```python
from build123d import *

# Parameters (mm, degrees)
CELL_BLOCK_SKETCH_W = 162.5
CELL_BLOCK_SKETCH_H = 305.12867922
BOSS_EXTRUDE1_DEPTH = 5
SKETCH3_W           = 7.5
SKETCH3_H           = 305.12867922
BOSS_EXTRUDE2_DEPTH = 5
HOLE_PATTERN_R      = 10.875
CUT_EXTRUDE1_DEPTH  = 5
SKETCH4_R           = 3.3
CUT_EXTRUDE2_DEPTH  = 5
SKETCH5_W           = 152.5
SKETCH5_H           = 25
BOSS_EXTRUDE3_DEPTH = 5
FILLET1_R           = 20


with BuildPart() as part:
    # Cell Block Sketch → Boss-Extrude1 (new body)
    with BuildSketch(Plane(origin=(0, 0, 0), x_dir=(1, 0, 0), z_dir=(0, 1, 0))):
        Rectangle(CELL_BLOCK_SKETCH_W, CELL_BLOCK_SKETCH_H)
    extrude(amount=BOSS_EXTRUDE1_DEPTH)

    # Sketch3 → Boss-Extrude2 (add)
    with BuildSketch(Plane(origin=(0, 0, 0), x_dir=(1, 0, 0), z_dir=(0, 1, 0))):
        with Locations((-85, 0)):
            Rectangle(SKETCH3_W, SKETCH3_H)
    boss_extrude2 = extrude(amount=BOSS_EXTRUDE2_DEPTH)

    # Mirror1: Boss-Extrude2 across plane
    add(boss_extrude2.mirror(Plane(origin=(0, 0, 0), x_dir=(0, 0, 1), z_dir=(1, 0, 0))))

    # Hole Pattern → Cut-Extrude1 (cut)
    with BuildSketch(Plane(origin=(0, 5, 0), x_dir=(1, 0, 0), z_dir=(0, 1, 0))):
        with Locations(Location((-70.375, -111.814056593, 0), (0, 0, 270))):
            Circle(HOLE_PATTERN_R)
        with Locations(Location((-58.9, -131.68933961, 0), (0, 0, 270))):
            Circle(HOLE_PATTERN_R)
        with Locations(Location((-70.375, -72.063490559, 0), (0, 0, 270))):
            Circle(HOLE_PATTERN_R)
        with Locations(Location((-58.9, -91.938773576, 0), (0, 0, 270))):
            Circle(HOLE_PATTERN_R)
        with Locations(Location((-70.375, -32.312924525, 0), (0, 0, 270))):
            Circle(HOLE_PATTERN_R)
        with Locations(Location((-58.9, -52.188207542, 0), (0, 0, 270))):
            Circle(HOLE_PATTERN_R)
        with Locations(Location((-70.375, 7.437641508, 0), (0, 0, 270))):
            Circle(HOLE_PATTERN_R)
        with Locations(Location((-58.9, -12.437641508, 0), (0, 0, 270))):
            Circle(HOLE_PATTERN_R)
        with Locations(Location((-70.375, 47.188207542, 0), (0, 0, 270))):
            Circle(HOLE_PATTERN_R)
        with Locations(Location((-58.9, 27.312924525, 0), (0, 0, 270))):
            Circle(HOLE_PATTERN_R)
        with Locations(Location((-70.375, 86.938773576, 0), (0, 0, 270))):
            Circle(HOLE_PATTERN_R)
        with Locations(Location((-58.9, 67.063490559, 0), (0, 0, 270))):
            Circle(HOLE_PATTERN_R)
        with Locations(Location((-70.375, 126.68933961, 0), (0, 0, 270))):
            Circle(HOLE_PATTERN_R)
        with Locations(Location((-58.9, 106.814056593, 0), (0, 0, 270))):
            Circle(HOLE_PATTERN_R)
        with Locations(Location((-47.425, -72.063490559, 0), (0, 0, 270))):
            Circle(HOLE_PATTERN_R)
        with Locations(Location((-35.95, -91.938773576, 0), (0, 0, 270))):
            Circle(HOLE_PATTERN_R)
        with Locations(Location((-47.425, -32.312924525, 0), (0, 0, 270))):
            Circle(HOLE_PATTERN_R)
        with Locations(Location((-35.95, -52.188207542, 0), (0, 0, 270))):
            Circle(HOLE_PATTERN_R)
        with Locations(Location((-47.425, 7.437641508, 0), (0, 0, 270))):
            Circle(HOLE_PATTERN_R)
        with Locations(Location((-35.95, -12.437641508, 0), (0, 0, 270))):
            Circle(HOLE_PATTERN_R)
        with Locations(Location((-47.425, 47.188207542, 0), (0, 0, 270))):
            Circle(HOLE_PATTERN_R)
        with Locations(Location((-35.95, 27.312924525, 0), (0, 0, 270))):
            Circle(HOLE_PATTERN_R)
        with Locations(Location((-47.425, 86.938773576, 0), (0, 0, 270))):
            Circle(HOLE_PATTERN_R)
        with Locations(Location((-35.95, 67.063490559, 0), (0, 0, 270))):
            Circle(HOLE_PATTERN_R)
        with Locations(Location((-47.425, 126.68933961, 0), (0, 0, 270))):
            Circle(HOLE_PATTERN_R)
        with Locations(Location((-35.95, 106.814056593, 0), (0, 0, 270))):
            Circle(HOLE_PATTERN_R)
        with Locations(Location((-24.475, -72.063490559, 0), (0, 0, 270))):
            Circle(HOLE_PATTERN_R)
        with Locations(Location((-13, -91.938773576, 0), (0, 0, 270))):
            Circle(HOLE_PATTERN_R)
        with Locations(Location((-24.475, -32.312924525, 0), (0, 0, 270))):
            Circle(HOLE_PATTERN_R)
        with Locations(Location((-13, -52.188207542, 0), (0, 0, 270))):
            Circle(HOLE_PATTERN_R)
        with Locations(Location((-24.475, 7.437641508, 0), (0, 0, 270))):
            Circle(HOLE_PATTERN_R)
        with Locations(Location((-13, -12.437641508, 0), (0, 0, 270))):
            Circle(HOLE_PATTERN_R)
        with Locations(Location((-24.475, 47.188207542, 0), (0, 0, 270))):
            Circle(HOLE_PATTERN_R)
        with Locations(Location((-13, 27.312924525, 0), (0, 0, 270))):
            Circle(HOLE_PATTERN_R)
        with Locations(Location((-24.475, 86.938773576, 0), (0, 0, 270))):
            Circle(HOLE_PATTERN_R)
        with Locations(Location((-13, 67.063490559, 0), (0, 0, 270))):
            Circle(HOLE_PATTERN_R)
        with Locations(Location((-24.475, 126.68933961, 0), (0, 0, 270))):
            Circle(HOLE_PATTERN_R)
        with Locations(Location((-13, 106.814056593, 0), (0, 0, 270))):
            Circle(HOLE_PATTERN_R)
        with Locations(Location((-47.425, -111.814056593, 0), (0, 0, 270))):
            Circle(HOLE_PATTERN_R)
        with Locations(Location((-35.95, -131.68933961, 0), (0, 0, 270))):
            Circle(HOLE_PATTERN_R)
        with Locations(Location((-24.475, -111.814056593, 0), (0, 0, 270))):
            Circle(HOLE_PATTERN_R)
        with Locations(Location((-13, -131.68933961, 0), (0, 0, 270))):
            Circle(HOLE_PATTERN_R)
        with Locations(Location((70.375, -131.68933961, 0), (0, 0, 270))):
            Circle(HOLE_PATTERN_R)
        with Locations(Location((58.9, -111.814056593, 0), (0, 0, 270))):
            Circle(HOLE_PATTERN_R)
        with Locations(Location((35.95, -111.814056593, 0), (0, 0, 270))):
            Circle(HOLE_PATTERN_R)
        with Locations(Location((47.425, -131.68933961, 0), (0, 0, 270))):
            Circle(HOLE_PATTERN_R)
        with Locations(Location((13, -111.814056593, 0), (0, 0, 270))):
            Circle(HOLE_PATTERN_R)
        with Locations(Location((24.475, -131.68933961, 0), (0, 0, 270))):
            Circle(HOLE_PATTERN_R)
        with Locations(Location((35.95, -72.063490559, 0), (0, 0, 270))):
            Circle(HOLE_PATTERN_R)
        with Locations(Location((47.425, -91.938773576, 0), (0, 0, 270))):
            Circle(HOLE_PATTERN_R)
        with Locations(Location((13, -72.063490559, 0), (0, 0, 270))):
            Circle(HOLE_PATTERN_R)
        with Locations(Location((24.475, -91.938773576, 0), (0, 0, 270))):
            Circle(HOLE_PATTERN_R)
        with Locations(Location((35.95, -32.312924525, 0), (0, 0, 270))):
            Circle(HOLE_PATTERN_R)
        with Locations(Location((47.425, -52.188207542, 0), (0, 0, 270))):
            Circle(HOLE_PATTERN_R)
        with Locations(Location((13, -32.312924525, 0), (0, 0, 270))):
            Circle(HOLE_PATTERN_R)
        with Locations(Location((24.475, -52.188207542, 0), (0, 0, 270))):
            Circle(HOLE_PATTERN_R)
        with Locations(Location((35.95, 7.437641508, 0), (0, 0, 270))):
            Circle(HOLE_PATTERN_R)
        with Locations(Location((47.425, -12.437641508, 0), (0, 0, 270))):
            Circle(HOLE_PATTERN_R)
        with Locations(Location((13, 7.437641508, 0), (0, 0, 270))):
            Circle(HOLE_PATTERN_R)
        with Locations(Location((24.475, -12.437641508, 0), (0, 0, 270))):
            Circle(HOLE_PATTERN_R)
        with Locations(Location((35.95, 47.188207542, 0), (0, 0, 270))):
            Circle(HOLE_PATTERN_R)
        with Locations(Location((47.425, 27.312924525, 0), (0, 0, 270))):
            Circle(HOLE_PATTERN_R)
        with Locations(Location((13, 47.188207542, 0), (0, 0, 270))):
            Circle(HOLE_PATTERN_R)
        with Locations(Location((24.475, 27.312924525, 0), (0, 0, 270))):
            Circle(HOLE_PATTERN_R)
        with Locations(Location((35.95, 86.938773576, 0), (0, 0, 270))):
            Circle(HOLE_PATTERN_R)
        with Locations(Location((47.425, 67.063490559, 0), (0, 0, 270))):
            Circle(HOLE_PATTERN_R)
        with Locations(Location((13, 86.938773576, 0), (0, 0, 270))):
            Circle(HOLE_PATTERN_R)
        with Locations(Location((24.475, 67.063490559, 0), (0, 0, 270))):
            Circle(HOLE_PATTERN_R)
        with Locations(Location((35.95, 126.68933961, 0), (0, 0, 270))):
            Circle(HOLE_PATTERN_R)
        with Locations(Location((47.425, 106.814056593, 0), (0, 0, 270))):
            Circle(HOLE_PATTERN_R)
        with Locations(Location((13, 126.68933961, 0), (0, 0, 270))):
            Circle(HOLE_PATTERN_R)
        with Locations(Location((24.475, 106.814056593, 0), (0, 0, 270))):
            Circle(HOLE_PATTERN_R)
        with Locations(Location((58.9, -72.063490559, 0), (0, 0, 270))):
            Circle(HOLE_PATTERN_R)
        with Locations(Location((70.375, -91.938773576, 0), (0, 0, 270))):
            Circle(HOLE_PATTERN_R)
        with Locations(Location((58.9, -32.312924525, 0), (0, 0, 270))):
            Circle(HOLE_PATTERN_R)
        with Locations(Location((70.375, -52.188207542, 0), (0, 0, 270))):
            Circle(HOLE_PATTERN_R)
        with Locations(Location((58.9, 7.437641508, 0), (0, 0, 270))):
            Circle(HOLE_PATTERN_R)
        with Locations(Location((70.375, -12.437641508, 0), (0, 0, 270))):
            Circle(HOLE_PATTERN_R)
        with Locations(Location((58.9, 47.188207542, 0), (0, 0, 270))):
            Circle(HOLE_PATTERN_R)
        with Locations(Location((70.375, 27.312924525, 0), (0, 0, 270))):
            Circle(HOLE_PATTERN_R)
        with Locations(Location((58.9, 86.938773576, 0), (0, 0, 270))):
            Circle(HOLE_PATTERN_R)
        with Locations(Location((70.375, 67.063490559, 0), (0, 0, 270))):
            Circle(HOLE_PATTERN_R)
        with Locations(Location((58.9, 126.68933961, 0), (0, 0, 270))):
            Circle(HOLE_PATTERN_R)
        with Locations(Location((70.375, 106.814056593, 0), (0, 0, 270))):
            Circle(HOLE_PATTERN_R)
    extrude(amount=-CUT_EXTRUDE1_DEPTH, mode=Mode.SUBTRACT)

    # Sketch4 → Cut-Extrude2 (cut)
    with BuildSketch(Plane(origin=(0, 5, 0), x_dir=(1, 0, 0), z_dir=(0, 1, 0))):
        with Locations(Location((-81.25, 104.43566039, 0), (0, 0, 270))):
            Circle(SKETCH4_R)
        with Locations(Location((-81.25, -15.06433961, 0), (0, 0, 270))):
            Circle(SKETCH4_R)
        with Locations(Location((-81.25, -134.56433961, 0), (0, 0, 270))):
            Circle(SKETCH4_R)
        with Locations(Location((81.25, -110.06433961, 0), (0, 0, 270))):
            Circle(SKETCH4_R)
        with Locations(Location((81.25, 9.43566039, 0), (0, 0, 270))):
            Circle(SKETCH4_R)
        with Locations(Location((81.25, 128.93566039, 0), (0, 0, 270))):
            Circle(SKETCH4_R)
    extrude(amount=-CUT_EXTRUDE2_DEPTH, mode=Mode.SUBTRACT)

    # Sketch5 → Boss-Extrude3 (add)
    with BuildSketch(Plane(origin=(0, 0, 0), x_dir=(1, 0, 0), z_dir=(0, 1, 0))):
        with Locations((-12.5, 165.06433961)):
            Rectangle(SKETCH5_W, SKETCH5_H)
    extrude(amount=BOSS_EXTRUDE3_DEPTH)

    # Fillet1
    fillet1_edges = [part.edges().sort_by_distance(p)[0] for p in [
        (-88.75, 2.5, -177.56433961),
    ]]
    fillet(fillet1_edges, radius=FILLET1_R)


solid = part.part
```
The model under review builds one solid part; all positions refer to its coordinate system, in mm. Coordinates: 2 decimals unless noted, no trailing zeros. Write each loop counter-clockwise with the first axis right and the second up, starting at its lowest first coordinate (ties: lowest second). Pieces come first, ordered by that corner, then holes.
1) We need section B-B on x = 41. Count the separate pieces of the cut face and the enclosed holes in it, then the cut area to 3 significant figures.
2) We need section A-A on z = 97. State the section outline as (x, y) points.
3) Clearance check with a flat-ended pin moving along its axis: pin 1 Ø13 at (x, z) = (-13, -67.06) entering from -Y. State where the tip first meets the part, or that it passes through.
4) The part is to be moulded in two halves that separate along Z. For faces 1 (the face through (-9.7, 2.5, 102.3)), 2 (the face through (-83, 2.5, -171.6)), 3 (the face through (-1, 5, -51)), say which applies: pulls with the +Z half, pulls with the -Z half, needs draft (parallel to the pull), parting line crosses it, or undercut.
Answer list:
1. separate pieces: 15
1. enclosed holes: 0
1. area: 362 mm2
2. outline: (-88.75, 0) - (-68.53, 0) - (-68.53, 5) - (-88.75, 5) - close; (-49.27, 0) - (-45.58, 0) - (-45.58, 5) - (-49.27, 5) - close; (-26.32, 0) - (-22.63, 0) - (-22.63, 5) - (-26.32, 5) - close; (-3.37, 0) - (14.85, 0) - (14.85, 5) - (-3.37, 5) - close; (34.1, 0) - (37.8, 0) - (37.8, 5) - (34.1, 5) - close; (57.05, 0) - (60.75, 0) - (60.75, 5) - (57.05, 5) - close; (80, 0) - (88.75, 0) - (88.75, 5) - (80, 5) - close
3. pin 1: passes through
4. face 1: undercut
4. face 2: pulls with the -Z half
4. face 3: needs draft
